Part model, mm, in its own coordinate system. A direction names the side the tool comes from. Give positions to 0.01 mm unless a question says otherwise; leave off trailing zeros. Write each loop counter-clockwise with the first axis right and the second up, starting at its lowest first coordinate (ties: lowest second). Pieces come first, ordered by that corner, then holes. Notation, with made-up numbers: M -28.75,69 L -17.75,69 A16 cw -17.75,96 Z; hole C 48.5,-26.5 d5. An arc over 180 degrees is marked long. Use CSV: the item, a comma, the result in double quotes. Start each with the question number.
Item 1: Pin check, flat tips, straight feed: pin 1 (2 mm diameter, centred on x = 16.5, z = -2.5, fed in from +Y); pin 2 (5 mm diameter, centred on x = -86, y = 5.5, fed in from -Z); pin 3 (12 mm diameter, centred on x = -3.5, z = -10.5, fed in from +Y). Stop position of each tip, or through.
Item 2: Drill centre lines: line 1 (Z direction, x = -82.5, y = -14); line 2 (Y direction, x = -118, z = 0); line 3 (Y direction, x = 36, z = -1). Where is each one in solid material? Low to high. Write a range as [from, to].
Item 3: Which spindle directions (+Z, -Z, +X, -X, +Y, -Y) get a long thin tool onto all of the face, cutting with end or side? Do faces 1 (the flat face through (-76.274, -38.9, 29.7)), 2 (the flat face through (-76.274, -26, -37)), 3 (the flat face through (-86, 25.463, 0)), 4 (the conical face through (-14.386, 8.431, 11.354)), 5 (the flat face through (-95.324, -38.9, 29.7)). Say none if no direction does.
Item 4: Cut at A-A (x = -52). List the corners of the cut face in (y, z).
Item 5: Mould opens along Z. For faces 6 (the cylindrical face through (-105.879, -35.371, -23.962)), 7 (the flat face through (-85.933, -32.714, 33.721)), 8 (the flat face through (-76.274, -38.9, -29.8)) say: released by +Z, released by -Z, zero draft, split by the parting line, or undercut.
from build123d import *

# Parameters (mm, degrees)
BOSS_EXTRUDE1_START = -1.185383
SKETCH2_W           = 19.05
SKETCH2_H           = 19.05
BOSS_EXTRUDE1_DEPTH = 1.185383
CIRPATTERN1_COUNT   = 3


with BuildPart() as part:
    # Sketch1 → Revolve1 (revolve)
    with BuildSketch(Plane.XY, mode=Mode.PRIVATE) as revolve1_sk:
        with BuildLine():
            Line((-14.12409666, 4.594554961), (-19.526618742, 9.997077044))
            ThreePointArc((-19.526618742, 9.997077044), (-29.623523347, 16.74361301), (-41.533634393, 19.112681394))
            Line((-41.533634393, 19.112681394), (-168.447274393, 19.112681394))
            Line((-168.447274393, 19.112681394), (-168.447274393, 25.462681394))
            Line((-168.447274393, 25.462681394), (-41.533634392, 25.462681394))
            ThreePointArc((-41.533634392, 25.462681394), (-29.623523346, 23.09361301), (-19.526618741, 16.347077044))
            Line((-19.526618741, 16.347077044), (-14.124096659, 10.944554962))
            ThreePointArc((-14.124096659, 10.944554962), (-8.491312805, 7.221332923), (-1.862483701, 5.937097346))
            ThreePointArc((-1.862483701, 5.937097346), (-0.908631777, 6.041561122), (-5.2e-08, 6.350000031))
            add(Edge.make_bspline(
                [(-5.2e-08, 6.350000031), (17.284276617, 14.409337901), (34.568553286, 21.376197316), (51.852829955, 27.377015197), (69.137106624, 32.507005795), (86.421383293, 36.843575686), (103.705659962, 40.451419137)],
                knots=[0.079490439, 0.079490439, 0.079490439, 0.079490439, 0.079490439, 0.079490439, 0.079490439, 0.916317313, 0.916317313, 0.916317313, 0.916317313, 0.916317313, 0.916317313, 0.916317313], degree=6))
            Line((103.705659962, 40.451419137), (103.705659962, 34.101419137))
            add(Edge.make_bspline(
                [(-5.3e-08, 3e-08), (17.284276616, 8.059337901), (34.568553285, 15.026197315), (51.852829954, 21.027015196), (69.137106623, 26.157005795), (86.421383292, 30.493575686), (103.705659962, 34.101419137)],
                knots=[0.079490439, 0.079490439, 0.079490439, 0.079490439, 0.079490439, 0.079490439, 0.079490439, 0.916317313, 0.916317313, 0.916317313, 0.916317313, 0.916317313, 0.916317313, 0.916317313], degree=6))
            ThreePointArc((-5.3e-08, 3e-08), (-0.908631778, -0.308438879), (-1.862483702, -0.412902654))
            ThreePointArc((-1.862483702, -0.412902654), (-8.491312805, 0.871332923), (-14.12409666, 4.594554961))
        make_face()
    revolve(revolve1_sk.sketch.rotate(Axis((-168.447274484, -13.3985, 0), (1, 0, 0)), 90), axis=Axis((-168.447274484, -13.3985, 0), (1, 0, 0)))

    # Sketch2 → Boss-Extrude1 (add)
    with BuildSketch(Plane(origin=(0, 25.462681394, 0), x_dir=(1, 0, 0), z_dir=(0, 1, 0)).offset(BOSS_EXTRUDE1_START)):
        with Locations((-85.799287115, 0)):
            Rectangle(SKETCH2_W, SKETCH2_H)
    boss_extrude1 = extrude(amount=BOSS_EXTRUDE1_DEPTH)

    # CirPattern1: Boss-Extrude1 ×3 about axis
    cirpattern1_axis = Axis((0, -13.3985, 0), (1, 0, 0))
    for i in range(1, CIRPATTERN1_COUNT):
        add(boss_extrude1.rotate(cirpattern1_axis, i * 360 / CIRPATTERN1_COUNT))


solid = part.part
Worked answers:
1,pin 1,"stops at y = 13.95"
1,pin 2,"stops at z = -35.23"
1,pin 3,"stops at y = 5.96"
2,line 1,"z = [-38.86, -32.51], [32.51, 38.86]"
2,line 2,"y = [-52.26, -45.91], [19.11, 25.46]"
2,line 3,"y = [-48.04, -41.69], [14.89, 21.25]"
3,face 1,"+Z, -Y"
3,face 2,"-Z, -Y"
3,face 3,"+Z, -Z, -X, +Y"
3,face 4,"none"
3,face 5,"+Z, -X, -Y"
4,outline,"C -13.4,0 d77.72; hole C -13.4,0 d65.02"
5,face 6,"undercut"
5,face 7,"released by +Z"
5,face 8,"zero draft"
